Autodesk Inventor part; units mm, degrees
ref_plane "YZ Plane" through (0, 0, 0) normal (1, 0, 0) x (0, 1, 0)
ref_plane "XZ Plane" through (0, 0, 0) normal (0, 1, 0) x (-1, 0, 0)
ref_plane "XY Plane" through (0, 0, 0) normal (0, 0, 1) x (1, 0, 0)
sketch "Sketch1" plane through (0, 0, 0) normal (0, 1, 0) x (-1, 0, 0)
  line L0 (-106.3625, -98.425) -> (106.3625, -98.425)
  line L1 (106.3625, -98.425) -> (106.3625, 98.425)
  line L2 (106.3625, 98.425) -> (-106.3625, 98.425)
  line L3 (-106.3625, 98.425) -> (-106.3625, -98.425)
  line L4 (-106.3625, -98.425) -> (106.3625, 98.425) construction
  line L5 (106.3625, -98.425) -> (-106.3625, 98.425) construction
  point P0 (0, 0)
  dimension "d0" = 212.725
  dimension "d1" = 196.85
extrude "Extrusion1" add sketch "Sketch1" against normal blind 72.05
sketch "Sketch2" plane through (-106.3625, 0, 98.425) normal (0, 0, 1) x (1, 0, 0)
  line L0 (0, -72.05) -> (212.725, -72.05)
  line L1 (11.906, -20) -> (200.819, -20)
  line L2 (200.819, -20) -> (200.819, -72.05)
  line L3 (200.819, -72.05) -> (11.906, -72.05)
  line L4 (11.906, -72.05) -> (11.906, -20)
  line L5 (0, 0) -> (212.725, 0)
  line L6 (0, 0) -> (0, -72.05)
  line L7 (212.725, 0) -> (212.725, -72.05)
  point P0 (106.3625, 0)
  point P1 (0, -36.025)
  point P2 (212.725, -36.025)
  dimension "d4" = 20
  dimension "d5" = 188.913
  dimension "d6" = 11.906
  dimension "d7" = 11.906
extrude "Extrusion2" cut sketch "Sketch2" against normal blind 172 contours L4 L1 L2 L0
sketch "Sketch3" plane through (-106.3625, 0, 98.425) normal (0, 0, 1) x (1, 0, 0)
  line L0 (11.906, -72.05) -> (11.906, -20)
  line L1 (11.906, -39.05) -> (21.906, -39.05)
  line L2 (21.906, -39.05) -> (21.906, -47.05)
  line L3 (21.906, -47.05) -> (11.906, -47.05)
  line L4 (11.906, -47.05) -> (11.906, -39.05)
  line L5 (200.819, -20) -> (200.819, -72.05)
  line L6 (200.819, -39.05) -> (190.819, -39.05)
  line L7 (190.819, -39.05) -> (190.819, -47.05)
  line L8 (190.819, -47.05) -> (200.819, -47.05)
  line L9 (200.819, -47.05) -> (200.819, -39.05)
  line L10 (11.906, -20) -> (200.819, -20)
  point P0 (106.3625, 0)
  point P1 (16.906, -39.05)
  point P2 (11.906, -47.05)
  dimension "d10" = 10
  dimension "d11" = 10
  dimension "d12" = 19.05
  dimension "d13" = 8
extrude "Extrusion3" add sketch "Sketch3" against normal blind 172
sketch "Sketch4" plane through (0, -72.05, 0) normal (0, -1, 0) x (1, 0, 0)
  line L0 (-106.3625, -98.425) -> (106.3625, -98.425)
  line L1 (-102.4, -98.425) -> (-65.887, -98.425)
  line L2 (-65.887, -98.425) -> (-65.887, -76.425)
  line L3 (-65.887, -76.425) -> (-102.4, -76.425)
  line L4 (-102.4, -76.425) -> (-102.4, -98.425)
  line L5 (65.887, -98.425) -> (102.4, -98.425)
  line L6 (102.4, -98.425) -> (102.4, -76.425)
  line L7 (102.4, -76.425) -> (65.887, -76.425)
  line L8 (65.887, -76.425) -> (65.887, -98.425)
  line L9 (-106.3625, 98.425) -> (-106.3625, -98.425)
  point P0 (0, 0)
  point P1 (102.4, -87.425)
  point P2 (65.887, -87.425)
  dimension "d16" = 36.513
  dimension "d17" = 36.513
  dimension "d18" = 22
  dimension "d19" = 22
  dimension "d20" = 131.774
  dimension "d21" = 3.9625
extrude "Extrusion4" cut sketch "Sketch4" against normal blind 5
properties material "Wood (Maple)"
Could you check a few things on this model? Use its own coordinates, in mm. A direction names the side the tool comes from. Coordinates: 2 decimals unless noted, no trailing zeros. Loops run counter-clockwise (first coordinate to the right, second up) from the corner with the lowest first, then second, coordinate; pieces in that order, holes last.
1. Imagine slicing it at A-A (y = -25). Please give me the cut outline in (x, z) (1 decimal).
2. I need wall thicknesses on L1, parallel to Y at x = -93, z = 13; L2, parallel to X at y = -22.5, z = 39.5; L3, parallel to X at y = -42, z = 62.5. Which ranges of each line are inside material? Lowest first, please.
3. Imagine slicing it at C-C (x = -76.5). Please give me the cut outline in (y, z) (3 decimals), and give its area (3 significant figures).
4. For P1, Ø1.5, axis at x = 33, y = -22.5, coming from the +Z side (3 decimals); P2, Ø5, axis at x = -79.5, z = -57.5, coming from the +Y side; P3, Ø12, axis at x = 77.5, z = -7, coming from the -Y side; P4, Ø6.5, axis at x = 86, z = -83, coming from the -Y side, each with a flat end and sliding along its axis, tell me the tip position at first contact or that it passes through.
5. Imagine slicing it at B-B (z = -7.5). Please give me the cut outline in (x, y), and give its area (3 significant figures).
6. Imagine slicing it at D-D (x = -11.5). Please give me the cut outline in (y, z) (3 decimals).
7. For faces 4 (the face through (-90, -39.05, 14)), 5 (the face through (24, -72.05, -80)), 6 (the face through (89, -47.05, 14)), 7 (the face through (-84, -70, -76.425)), 8 (the face through (1, 0, 1)), which set-ups out of +Z, -Z, +X, -X, +Y, -Y let a thin tool reach every point of the face, with its end or its side?
8. We'd pull the mould along X, two halves only. Please class faces 1 (the face through (106.362, -36, 1)), 2 (the face through (-25.1, -19.5, 98.425)), 3 (the face through (84, -70, -76.425)): released by +X, released by -X, zero draft, split by the parting line, or undercut.
Computed values:
1. outline: (-106.4, -98.4) - (106.4, -98.4) - (106.4, 98.4) - (94.5, 98.4) - (94.5, -73.6) - (-94.5, -73.6) - (-94.5, 98.4) - (-106.4, 98.4) - close
2. L1: y = -47.05 to -39.05, -20 to 0
2. L2: x = -106.36 to -94.46, 94.46 to 106.36
2. L3: x = -106.36 to -84.46, 84.46 to 106.36
3. outline: (-72.05, -76.425) - (-67.05, -76.425) - (-67.05, -98.425) - (0, -98.425) - (0, 98.425) - (-20, 98.425) - (-20, -73.575) - (-72.05, -73.575) - close
3. area: 5,120 mm2
4. P1: stops at z = -73.575
4. P2: stops at y = 0
4. P3: stops at y = -20
4. P4: stops at y = -67.05
5. outline: (-106.36, -72.05) - (-94.46, -72.05) - (-94.46, -47.05) - (-84.46, -47.05) - (-84.46, -39.05) - (-94.46, -39.05) - (-94.46, -20) - (94.46, -20) - (94.46, -39.05) - (84.46, -39.05) - (84.46, -47.05) - (94.46, -47.05) - (94.46, -72.05) - (106.36, -72.05) - (106.36, 0) - (-106.36, 0) - close
5. area: 5,650 mm2
6. outline: (-72.05, -98.425) - (0, -98.425) - (0, 98.425) - (-20, 98.425) - (-20, -73.575) - (-72.05, -73.575) - close
7. face 4: +Z
7. face 5: +Z, -Z, +X, -X, -Y
7. face 6: +Z, -Y
7. face 7: -Z, -Y
7. face 8: +Z, -Z, +X, -X, +Y
8. face 1: released by +X
8. face 2: zero draft
8. face 3: undercut
